Can you work these out from the model? Positions are in its coordinate system, mm. Face numbers are marked on the shaded views. A direction names the side the tool comes from. Give positions to 0.01 mm unless a question says otherwise; leave off trailing zeros. Write each loop counter-clockwise with the first axis right and the second up, starting at its lowest first coordinate (ties: lowest second). Pieces come first, ordered by that corner, then holes. Notation, with made-up numbers: (9.5, 60.5) - (61.5, 60.5) arc R33 cw to (61.5, 90.5) - close; hole circle Ø5 at (13.5, 88.5). An arc over 180 degrees is marked (long way). Return JSON: item names as keys, results as strings. Group by question number.
from build123d import *

# Parameters (mm, degrees)
F0_W        = 40
F0_H        = 40
F0_R        = 1.75
F0_R_2      = 17.5
F1_DEPTH    = 2
F2_R        = 5
F3_DEPTH    = 15
F4_W        = 8
F4_H        = 15
F5_DEPTH    = 15
F6_T1_DEPTH = 33
F6_T3_DEPTH = 42
F6_T5_DEPTH = 27


# Not quite as in the source:
# - a fillet or chamfer that OpenCascade refuses, or shapes differently, is made with other operations: its cross-section is extruded or revolved along the edge and cut away or added


with BuildPart() as f1:
    # F0 (on Top) → F1 (new body)
    with BuildSketch(Plane.XY):
        with Locations((9.0173190544, -26.0413483679)):
            Rectangle(F0_W, F0_H)
        with Locations((-7.2326809456, -42.2913483679)):
            Circle(F0_R, mode=Mode.SUBTRACT)
        with Locations((25.2673190544, -42.2913483679)):
            Circle(F0_R, mode=Mode.SUBTRACT)
        with Locations((9.0173190544, -26.0413483679)):
            Circle(F0_R_2, mode=Mode.SUBTRACT)
        with Locations((-7.2326809456, -9.7913483679)):
            Circle(F0_R, mode=Mode.SUBTRACT)
        with Locations((25.2673190544, -9.7913483679)):
            Circle(F0_R, mode=Mode.SUBTRACT)
    extrude(amount=F1_DEPTH)

    # F2
    f2_edges = [f1.edges().sort_by_distance(p)[0] for p in [
        (29.017319, -46.041348, 1),
        (29.017319, -6.041348, 1),
        (-10.982681, -46.041348, 1),
        (-10.982681, -6.041348, 1),
    ]]
    fillet(f2_edges, radius=F2_R)

    # F3 (add): a face of the model
    f3_faces = [f1.faces().sort_by_distance(p)[0] for p in [
        (29.0173190544, -26.0413483679, 1),
    ]]
    extrude(f3_faces, amount=F3_DEPTH)

    # F4 (on face) → F5 (join)
    with BuildSketch(Plane.XY.offset(2)):
        with Locations((40.0173190544, -18.5413483679)):
            Rectangle(F4_W, F4_H)
    extrude(amount=F5_DEPTH)

    # F6: fillet of radius 5 on 5 edges, made by hand

    # F6_s2 → F6_t1 (cut)
    with BuildSketch(Plane.YZ.offset(23.5173190544)):
        with BuildLine():
            ThreePointArc((-21.0413483679, 17), (-24.5768822739, 15.5355339059), (-26.0413483679, 12))
            Line((-26.0413483679, 12), (-26.0413483679, 17))
            Line((-26.0413483679, 17), (-21.0413483679, 17))
        make_face()
        with BuildLine():
            ThreePointArc((-16.0413483679, 17), (-12.505814462, 15.5355339059), (-11.0413483679, 12))
            Line((-11.0413483679, 12), (-11.0413483679, 17))
            Line((-11.0413483679, 17), (-16.0413483679, 17))
        make_face()
    extrude(amount=F6_T1_DEPTH, mode=Mode.SUBTRACT)

    # F6_s4 → F6_t3 (cut)
    with BuildSketch(Plane.XY.offset(-12.5)):
        with BuildLine():
            ThreePointArc((44.0173190544, -16.0413483679), (42.5528529604, -12.505814462), (39.0173190544, -11.0413483679))
            Line((39.0173190544, -11.0413483679), (44.0173190544, -11.0413483679))
            Line((44.0173190544, -11.0413483679), (44.0173190544, -16.0413483679))
        make_face()
    extrude(amount=F6_T3_DEPTH, mode=Mode.SUBTRACT)

    # F6_s6 → F6_t5 (cut)
    with BuildSketch(Plane.XY.offset(-12.5)):
        with BuildLine():
            ThreePointArc((39.0173190544, -41.0413483679), (42.5528529604, -39.5768822739), (44.0173190544, -36.0413483679))
            Line((44.0173190544, -36.0413483679), (44.0173190544, -41.0413483679))
            Line((44.0173190544, -41.0413483679), (39.0173190544, -41.0413483679))
        make_face()
    extrude(amount=F6_T5_DEPTH, mode=Mode.SUBTRACT)


solid = f1.part
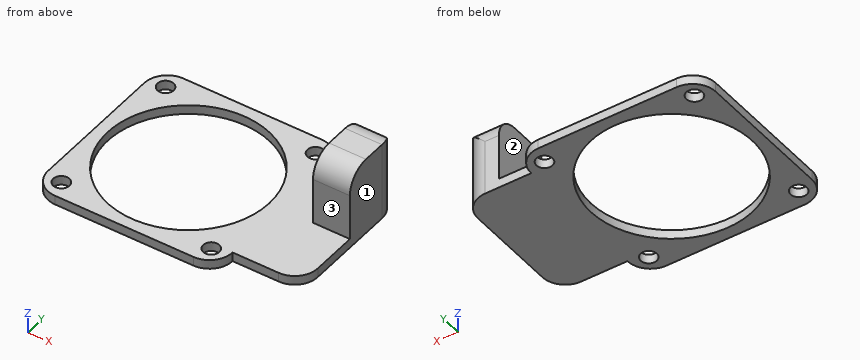
1) Imagine slicing it at B-B, the plane y = -17. Write out the boundary of the cut face in (x, z), and give its area (3 significant figures).
2) Imagine slicing it at C-C, the plane z = 5.5. Write out the boundary of the cut face in (x, y), and give its area (3 significant figures).
3) On a 3-axis mill with a long thin cutter (end or side, diameter ignored), from which of +Z, -Z, +X, -X, +Y, -Y can I reach the whole of each face in a straight line? I mean the marked faces 1, 2 and 3. Say none if no direction works.
4) Imagine slicing it at D-D, the plane y = -37.5. Write out the boundary of the cut face in (x, z), and give its area (3 significant figures).
5) Will these pins go through, and if not, where does the flat tip stop? pin 1 Ø3 at (x, z) = (35.5, 11) entering from +Y; pin 2 Ø1 at (x, z) = (35.5, 0.5) entering from -Y; pin 3 Ø6 at (y, z) = (-31, 4.5) entering from +X; pin 4 Ø2.5 at (x, z) = (41.5, 5) entering from -Y.
6) I need wall thicknesses on line 1 along Y through (x, z) = (9.5, 1); line 2 along Z through (x, y) = (29.5, -18); line 3 along X through (y, z) = (-24, 9.25). Which ranges of each line are inside material? Lowest first, please.
7) Imagine slicing it at A-A, the plane x = -1. Write out the boundary of the cut face in (y, z).
Resolved:
{
 "1": {"outline": "(-10.98, 0) - (-5.97, 0) - (-5.97, 2) - (-10.98, 2) - close; (24, 0) - (44.02, 0) - (44.02, 17) - (36.02, 17) - (36.02, 2) - (24, 2) - close", "area": "170 mm^2"},
 "2": {"outline": "(36.02, -26.04) - (44.02, -26.04) - (44.02, -16.04) arc R5 ccw to (39.02, -11.04) - (36.02, -11.04) - close", "area": "115 mm^2"},
 "3": {"face 1": "+Z, -Z, +X, +Y, -Y", "face 2": "+Z, -X, +Y, -Y", "face 3": "+Z, +X, -X, -Y"},
 "4": {"outline": "(-10.98, 0) - (-4.21, 0) - (-4.21, 2) - (-10.98, 2) - close; (22.24, 0) - (43.8, 0) - (43.8, 2) - (22.24, 2) - close", "area": "56.7 mm^2"},
 "5": {"pin 1": "y = -11.04", "pin 2": "y = -41.04", "pin 3": "x = 44.02", "pin 4": "y = -26.04"},
 "6": {"line 1": "-46.04 to -43.53, -8.55 to -6.04", "line 2": "0 to 2", "line 3": "36.02 to 44.02"},
 "7": {"outline": "(-46.04, 0) - (-40.39, 0) - (-40.39, 2) - (-46.04, 2) - close; (-11.69, 0) - (-6.04, 0) - (-6.04, 2) - (-11.69, 2) - close"}
}
